Could you check a few things on this model? Use its own coordinates, in mm. A direction names the side the tool comes from. Coordinates: 2 decimals unless noted, no trailing zeros. Write each loop counter-clockwise with the first axis right and the second up, starting at its lowest first coordinate (ties: lowest second). Pieces come first, ordered by that corner, then holes. Notation, with made-up numbers: (-40, 51.5) - (-27, 51.5) arc R21 ccw to (-27, 80.5) - close; hole circle Ø7 at (12.5, 80). An arc over 180 degrees is marked (long way). Write item = value, one per line. Start each with the question number.
Autodesk Inventor part; units mm, degrees
ref_plane "YZ Plane" through (0, 0, 0) normal (1, 0, 0) x (0, 1, 0)
ref_plane "XZ Plane" through (0, 0, 0) normal (0, 1, 0) x (-1, 0, 0)
ref_plane "XY Plane" through (0, 0, 0) normal (0, 0, 1) x (1, 0, 0)
ref_plane "Plano de trabalho2" through (-4.1, 8.25, 200) normal (0, 0, 1) x (1, 0, 0)
sketch "Esboço2" plane through (-4.1, 8.25, 200) normal (0, 0, 1) x (1, 0, 0)
  line L0 (-6.9, 3.8107) -> (-6.9, 10.25)
  line L1 (-6.9, 10.25) -> (-6.9, 3.8107)
  line L2 (12.7893, 1.5) -> (-4.5893, 1.5)
  line L3 (-6.9, 3.8107) -> (-4.5893, 1.5)
  line L4 (-4.5893, 1.5) -> (12.7893, 1.5)
  line L5 (12.7893, 1.5) -> (15.1, 3.8107)
  line L6 (15.1, 10.25) -> (15.1, 3.8107)
  line L7 (15.1, 3.8107) -> (15.1, 10.25)
  line L8 (10.7, 10.25) -> (15.1, 10.25)
  line L9 (15.1, 10.25) -> (10.7, 10.25)
  line L10 (9.7, 7.75) -> (9.7, 9.25)
  line L11 (10.7, 10.25) -> (9.7, 9.25)
  line L12 (9.7, 9.25) -> (9.7, 7.75)
  line L13 (9.7, 7.75) -> (8.2, 7.75)
  line L14 (15.1, 11.75) -> (8.2, 11.75)
  line L15 (8.2, 7.75) -> (8.2, 11.75)
  line L16 (0, 7.75) -> (0, 11.75)
  line L17 (8.2, 11.75) -> (0, 11.75)
  line L18 (0, 11.75) -> (0, 7.75)
  line L19 (0, 7.75) -> (-1.5, 7.75)
  line L20 (-2.5, 10.25) -> (-1.5, 9.25)
  line L21 (-1.5, 7.75) -> (-1.5, 9.25)
  line L22 (-1.5, 9.25) -> (-2.5, 10.25)
  line L23 (-2.5, 10.25) -> (-6.9, 10.25)
  point P0 (4.1, -8.25)
extrude "Extrusão1" add sketch "Esboço2" along normal blind 10
ref_plane "Plano de trabalho5" through (-4.1, 20, 200) normal (0, 1, 0) x (1, 0, 0)
sketch "Esboço3" plane through (-4.1, 20, 200) normal (0, 1, 0) x (1, 0, 0)
  circle A0 centre (4.1, -5) radius 2.5
  line L0 (19.5, 0) -> (-11.3, 0)
  line L1 (15.1, 0) -> (15.1, -10)
  point P0 (4.1, 200)
  dimension "d2" = 5
  dimension "d3" = 5
  dimension "d4" = 11
hole "Furo1" at (0, 20, 205) direction (0, -1, 0) diameter 5 depth 20 tip angle 118
properties part number "Pecinha do perfil_CPY" material "Alumínio"
1) Suppose I cut it at B-B on y = 16.75. Please give me the cut outline in (x, z), plus the area to 3 significant figures.
2) If I drill on probe 1 along X at (y, z) = (16.5, 205); probe 2 along Z at (x, y) = (0, 17.5); probe 3 along X at (y, z) = (14.75, 205), over which ranges is the centre line in solid material (lowest first)? Write a range as [from, to].
3) Suppose I cut it at D-D on y = 14. Please give me the cut outline in (x, z), plus the area to 3 significant figures.
4) For P1, Ø1.3, axis at x = -8.5, z = 207, coming from the +Y side; P2, Ø1.6, axis at x = -5, z = 203, coming from the +Y side, each with a flat end and sliding along its axis, tell me the tip position at first contact or that it passes through.
5) Which directions (+Z, -Z, +X, -X, +Y, -Y) give clear straight access to the entire face, cutting with the end or side of a thin tool? Please do faces 5 (the flat face through (-9, 18.5, 205)), 6 (the flat face through (9, 18.5, 205)), 7 (the flat face through (-5, 16, 205)), 8 (the flat face through (11, 15, 205)).
6) Suppose I cut it at A-A on z = 205. Please give me the cut outline in (x, y).
7) Suppose I cut it at C-C on x = 0. Please give me the cut outline in (y, z), plus the area to 4 significant figures.
8) Thinking about a two-plate mould opening in Z: for faces 1 (the flat face through (0, 15, 210)), 2 (the flat face through (4.1, 18, 205)), 3 (the flat face through (0, 15, 200)), 4 (the cylindrical face through (-0.751, 14.803, 207.385)), which applies, +Z half, -Z half, draft (parallel to the pull), parting line (faces both ways), or undercut?
Reply:
q1.outline = (-11, 200) - (-5.6, 200) - (-5.6, 210) - (-11, 210) - close; (-4.1, 200) - (4.1, 200) - (4.1, 210) - (-4.1, 210) - close; (5.6, 200) - (11, 200) - (11, 210) - (5.6, 210) - close; hole circle Ø5 at (0, 205)
q1.area = 170 mm^2
q2.probe_1 = [-11, -5.6], [-4.1, -2.5], [2.5, 4.1], [5.6, 11]
q2.probe_2 = [200, 202.5], [207.5, 210]
q2.probe_3 = [-11, -2.5], [2.5, 11]
q3.outline = (-11, 200) - (11, 200) - (11, 210) - (-11, 210) - close; hole circle Ø5 at (0, 205)
q3.area = 200 mm^2
q4.P1 = 18.5
q4.P2 = 17.7
q5.face_5 = +Z, -Z, -X, +Y
q5.face_6 = +Z, -Z, +X, +Y
q5.face_7 = +Z, -Z, +Y
q5.face_8 = +Z, -Z, +X, +Y, -Y
q6.outline = (-11, 12.06) - (-8.69, 9.75) - (-2.5, 9.75) - (-2.5, 20) - (-4.1, 20) - (-4.1, 16) - (-5.6, 16) - (-5.6, 17.5) - (-6.6, 18.5) - (-11, 18.5) - close; (2.5, 9.75) - (8.69, 9.75) - (11, 12.06) - (11, 18.5) - (6.6, 18.5) - (5.6, 17.5) - (5.6, 16) - (4.1, 16) - (4.1, 20) - (2.5, 20) - close
q7.outline = (9.75, 200) - (20, 200) - (20, 202.5) - (9.75, 202.5) - close; (9.75, 207.5) - (20, 207.5) - (20, 210) - (9.75, 210) - close
q7.area = 51.25 mm^2
q8.face_1 = +Z half
q8.face_2 = draft
q8.face_3 = -Z half
q8.face_4 = undercut
